The listing builds one solid part. Answer for the finished solid, in the listing's coordinates (mm). A direction names the side the tool comes from. Give positions to 0.01 mm unless a question says otherwise; leave off trailing zeros. Write each loop counter-clockwise with the first axis right and the second up, starting at its lowest first coordinate (ties: lowest second). Pieces come first, ordered by that corner, then holes. Notation, with made-up numbers: (-5, 82.5) -> (43, 82.5) arc R28 ccw to (43, 108.5) -> close; hole circle Ø4 at (59.25, -13.5). An arc over 180 degrees is marked (long way). One line per question, with ' | ' between items.
from build123d import *

# Parameters (mm, degrees)
SKETCH1_R                 = 20
BOSS_EXTRUDE1_DEPTH       = 6
CUT_EXTRUDE1_DEPTH        = 29.91366459
CIRPATTERN1_COUNT         = 3
SKETCH3_W                 = 7
SKETCH3_H                 = 20
BOSS_EXTRUDE2_DEPTH       = 25
SKETCH4_W                 = 9.525
SKETCH4_H                 = 12
CUT_EXTRUDE2_DEPTH        = 44.7407133
FILLET1_R                 = 1
FILLET2_R                 = 3
CUT_EXTRUDE3_DEPTH        = 38.749172176
M4X0_7_TAPPED_HOLE1_D     = 3.3
M4X0_7_TAPPED_HOLE1_DEPTH = 8.1
M4X0_7_TAPPED_HOLE1_TIP   = 0.991420021
FILLET3_R                 = 5


with BuildPart() as part:
    # Sketch1 → Boss-Extrude1 (new body)
    with BuildSketch(Plane(origin=(0, 0, 0), x_dir=(1, 0, 0), z_dir=(0, 1, 0))):
        with Locations(Location((0, 0, 0), (0, 0, 270))):
            Circle(SKETCH1_R)
    extrude(amount=BOSS_EXTRUDE1_DEPTH)

    # Sketch2 → Cut-Extrude1 (cut, through all)
    with BuildSketch(Plane(origin=(0, 6, 0), x_dir=(1, 0, 0), z_dir=(0, 1, 0))):
        with BuildLine():
            ThreePointArc((0, 17), (-2, 15), (0, 13))
            ThreePointArc((0, 13), (6.5, 11.258330249), (11.258330249, 6.5))
            ThreePointArc((11.258330249, 6.5), (13.990381057, 5.767949192), (14.722431864, 8.5))
            ThreePointArc((14.722431864, 8.5), (8.5, 14.722431864), (0, 17))
        make_face()
    cut_extrude1 = extrude(amount=-CUT_EXTRUDE1_DEPTH, mode=Mode.SUBTRACT)

    # CirPattern1: Cut-Extrude1 ×3 about axis
    cirpattern1_axis = Axis((0, 0, 0), (0, 1, 0))
    for i in range(1, CIRPATTERN1_COUNT):
        add(cut_extrude1.rotate(cirpattern1_axis, i * 360 / CIRPATTERN1_COUNT), mode=Mode.SUBTRACT)

    # Sketch3 → Boss-Extrude2 (add)
    with BuildSketch(Plane(origin=(0, 6, 0), x_dir=(1, 0, 0), z_dir=(0, 1, 0))):
        Rectangle(SKETCH3_W, SKETCH3_H)
    extrude(amount=BOSS_EXTRUDE2_DEPTH)

    # Sketch4 → Cut-Extrude2 (cut, through all)
    with BuildSketch(Plane(origin=(3.5, 0, 0), x_dir=(0, 0, -1), z_dir=(1, 0, 0))):
        with Locations((0, 25)):
            Rectangle(SKETCH4_W, SKETCH4_H)
    extrude(amount=-CUT_EXTRUDE2_DEPTH, mode=Mode.SUBTRACT)

    # Fillet1
    fillet1_edges = [part.edges().sort_by_distance(p)[0] for p in [
        (0, 6, 10),
        (0, 6, -10),
    ]]
    fillet(fillet1_edges, radius=FILLET1_R)

    # Fillet2
    fillet2_edges = [part.edges().sort_by_distance(p)[0] for p in [
        (-3.5, 6, 0),
    ]]
    fillet(fillet2_edges, radius=FILLET2_R)
    fillet2_2_edges = [part.edges().sort_by_distance(p)[0] for p in [
        (3.5, 6, 0),
    ]]
    fillet(fillet2_2_edges, radius=FILLET2_R)

    # Sketch5 → Cut-Extrude3 (cut, through all)
    with BuildSketch(Plane(origin=(0, 6, 0), x_dir=(1, 0, 0), z_dir=(0, 1, 0))):
        with BuildLine():
            Line((-9.5, 13), (-3.5, 13))
            Line((-3.5, 13), (-3.5, 8))
            ThreePointArc((-3.5, 8), (-4.964466094, 4.464466094), (-8.5, 3))
            Line((-8.5, 3), (-9.5, 3))
            Line((-9.5, 3), (-9.5, 13))
        make_face()
        with BuildLine():
            Line((9.5, 3), (8.5, 3))
            ThreePointArc((8.5, 3), (4.964466094, 4.464466094), (3.5, 8))
            Line((3.5, 8), (3.5, 13))
            Line((3.5, 13), (9.5, 13))
            Line((9.5, 13), (9.5, 3))
        make_face()
        with BuildLine():
            Line((9.5, -13), (9.5, -3))
            Line((9.5, -3), (8.5, -3))
            ThreePointArc((8.5, -3), (4.964466094, -4.464466094), (3.5, -8))
            Line((3.5, -8), (3.5, -13))
            Line((3.5, -13), (9.5, -13))
        make_face()
        with BuildLine():
            Line((-3.5, -13), (-3.5, -8))
            ThreePointArc((-3.5, -8), (-4.964466094, -4.464466094), (-8.5, -3))
            Line((-8.5, -3), (-9.5, -3))
            Line((-9.5, -3), (-9.5, -13))
            Line((-9.5, -13), (-3.5, -13))
        make_face()
    extrude(amount=CUT_EXTRUDE3_DEPTH, mode=Mode.SUBTRACT)

    # M4x0.7 Tapped Hole1
    with Locations(Plane(origin=(0, 19, 0), x_dir=(-1, 0, 0), z_dir=(0, 1, 0))):
        with Locations((0, 0)):
            Hole(M4X0_7_TAPPED_HOLE1_D / 2, depth=M4X0_7_TAPPED_HOLE1_DEPTH)
            with Locations((0, 0, -(M4X0_7_TAPPED_HOLE1_DEPTH + M4X0_7_TAPPED_HOLE1_TIP / 2))):  # 118° drill point
                Cone(0, M4X0_7_TAPPED_HOLE1_D / 2, M4X0_7_TAPPED_HOLE1_TIP, mode=Mode.SUBTRACT)

    # Fillet3
    fillet3_edges = [part.edges().sort_by_distance(p)[0] for p in [
        (0, 31, 10),
        (0, 31, -10),
    ]]
    fillet(fillet3_edges, radius=FILLET3_R)


solid = part.part
Item 1: Find section B-B (x = 13.5). Write down the section's boundary in (y, z), then the cut area to 3 significant figures.
Answers below:
outline: (0, -14.76) -> (6, -14.76) -> (6, -10.33) -> (0, -10.33) -> close; (0, -5.57) -> (6, -5.57) -> (6, 5.57) -> (0, 5.57) -> close; (0, 10.33) -> (6, 10.33) -> (6, 14.76) -> (0, 14.76) -> close | area: 120 mm²
Item 2: Find section D-D (y = 28). Write down the section's boundary in (x, z), then the cut area to 3 significant figures.
Answers below:
outline: (-3.5, -9.58) -> (3.5, -9.58) -> (3.5, -4.76) -> (-3.5, -4.76) -> close; (-3.5, 4.76) -> (3.5, 4.76) -> (3.5, 9.58) -> (-3.5, 9.58) -> close | area: 67.5 mm²
Item 3: A tool of negligible diameter and unlimited length cuts with its end or side. For faces 4 (the face through (-17, 3, 0)), 5 (the face through (0, 16, 10)), 6 (the face through (-3.744, 6.812, -6.456)), from which of +Z, -Z, +X, -X, +Y, -Y can it reach the whole face along a straight path? Write none if from no direction.
Answers below:
face 4: +Y, -Y | face 5: +Z, +X, -X, +Y | face 6: -Z, -X, +Y
Item 4: Flat-ended cylindrical pins translate along their axes: pin 1 (11 mm diameter, centred on y = 17, z = 1.5, fed in from -X); pin 2 (10 mm diameter, centred on y = 7, z = 8.5, fed in from -X); pin 3 (3.5 mm diameter, centred on x = 0, z = -1, fed in from +Y). Find the tip coordinate at first contact, or state that the pin passes through.
Answers below:
pin 1: x = -3.5 | pin 2: x = -19.67 | pin 3: y = 19
Item 5: Consider line 1 (X direction, y = 15.5, z = 0); line 2 (Z direction, x = 0, y = 14.5); line 3 (X direction, y = 4.5, z = 9). Determine where each line is inside the solid, lowest interval first. Write a range as [from, to].
Answers below:
line 1: [-3.5, -1.65], [1.65, 3.5] | line 2: [-10, -1.65], [1.65, 10] | line 3: [-17.86, -14.31], [-11.67, 9.38], [14.42, 17.86]
Item 6: Find section C-C (z = -15). Write down the section's boundary in (x, y), then the cut area to 3 significant figures.
Answers below:
outline: (-13.23, 0) -> (-2, 0) -> (-2, 6) -> (-13.23, 6) -> close; (8, 0) -> (13.23, 0) -> (13.23, 6) -> (8, 6) -> close | area: 98.7 mm²
Item 7: Find section A-A (y = 18). Write down the section's boundary in (x, z), then the cut area to 3 significant figures.
Answers below:
outline: (-3.5, -10) -> (3.5, -10) -> (3.5, 10) -> (-3.5, 10) -> close; hole circle Ø3.3 at (0, 0) | area: 131 mm²
Item 8: Determine the mould class of faces 1 (the face through (2, 19, -1)), 2 (the face through (3.5, 18, 0)), 3 (the face through (0.049, 6.285, 10.301)) for opening direction Z: pulls with the +Z half, pulls with the -Z half, needs draft (parallel to the pull), parting line crosses it, or undercut.
Answers below:
face 1: undercut | face 2: needs draft | face 3: pulls with the +Z half
